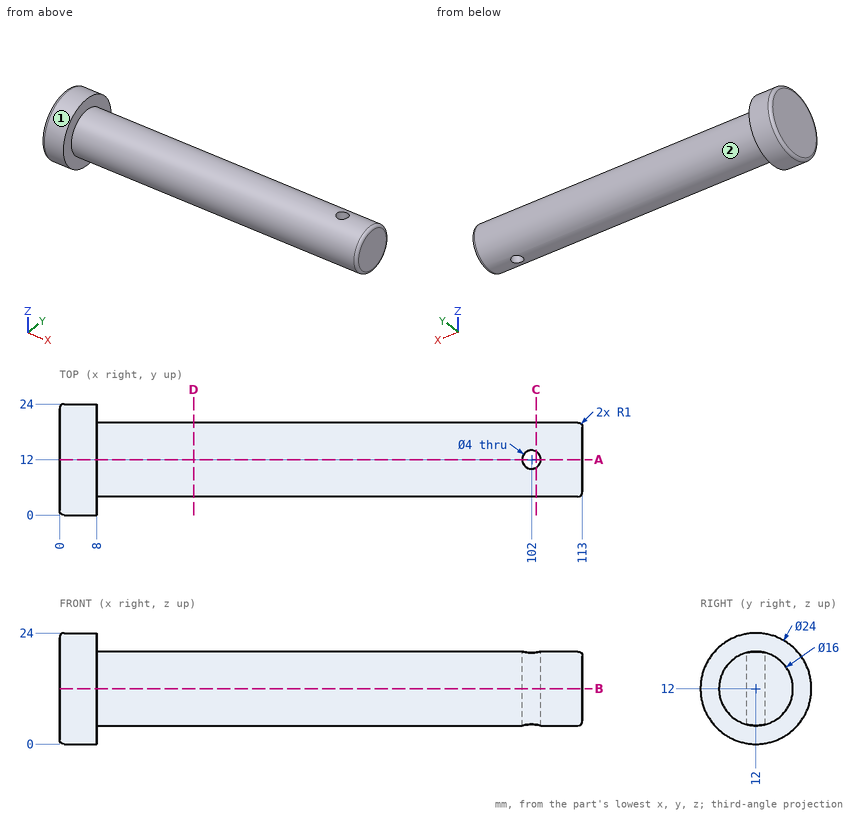
Here's the drawing with two shaded views (mm, measured from the low corner). I have some questions. A direction names the side the tool comes from. Give positions to 0.01 mm unless a question says otherwise; leave off trailing zeros. Write each loop counter-clockwise with the first axis right and the second up, starting at its lowest first coordinate (ties: lowest second). Pieces come first, ordered by that corner, then holes. Notation, with made-up numbers: (24, 77.25) -> (60, 77.25) arc R22 cw to (60, 85.25) -> close; hole circle Ø11 at (88, 57.25). An arc over 180 degrees is marked (long way). Use one line per item in the form item = value.
1) Suppose I cut it at D-D (x = 29). Please give me the cut outline in (y, z), and give its area (3 significant figures).
Verdict:
outline = circle Ø16 at (12, 12)
area = 201 mm2
2) Suppose I cut it at B-B (z = 12). Please give me the cut outline in (x, y).
Verdict:
outline = (0, 1) arc R1 ccw to (1, 0) -> (8, 0) -> (8, 4) -> (112, 4) arc R1 ccw to (113, 5) -> (113, 19) arc R1 ccw to (112, 20) -> (8, 20) -> (8, 24) -> (1, 24) arc R1 ccw to (0, 23) -> close; hole circle Ø4 at (102, 12)
3) I'm going to push flat-ended pins straight in: pin 1 (5 mm diameter, centred on x = 34, y = 16, fed in from -Z); pin 2 (8 mm diameter, centred on x = 99, z = 13, fed in from -Y); pin 3 (5 mm diameter, centred on x = 59.5, y = 7.5, fed in from +Z). Where does each tip first touch, or does it pass through?
Verdict:
pin_1 = 4.14
pin_2 = 4
pin_3 = 19.75
4) Suppose I cut it at A-A (y = 12). Please give me the cut outline in (x, z).
Verdict:
outline = (0, 1) arc R1 ccw to (1, 0) -> (8, 0) -> (8, 4) -> (100, 4) -> (100, 20) -> (8, 20) -> (8, 24) -> (1, 24) arc R1 ccw to (0, 23) -> close; (104, 4) -> (112, 4) arc R1 ccw to (113, 5) -> (113, 19) arc R1 ccw to (112, 20) -> (104, 20) -> close
5) If I drill on L1, parallel to X at y = 12, z = 8.25; L2, parallel to Y at x = 102, z = 8.25; L3, parallel to Z at x = 71, y = 11.5, over which ranges is the centre line in solid material (lowest first)? Write a range as [from, to].
Verdict:
L1 = [0, 100], [104, 113]
L2 = [4.93, 10], [14, 19.07]
L3 = [4.02, 19.98]
6) On a 3-axis mill with a long thin cutter (end or side, diameter ignored), from which of +Z, -Z, +X, -X, +Y, -Y can I reach the whole of each face in a straight line? I mean the marked faces 1 and 2. Say none if no direction works.
Verdict:
face_1 = +X, -X
face_2 = +X
7) Suppose I cut it at C-C (x = 103). Please give me the cut outline in (y, z).
Verdict:
outline = (10.27, 4.19) -> (10.27, 19.81) arc R8 ccw to start; (13.73, 4.19) arc R8 ccw to (13.73, 19.81) -> close
